```python
from build123d import *

# Parameters (mm, degrees)
SKETCH053_R         = 4
PAD024_DEPTH        = 134.8
SKETCH063_R         = 3.3
PAD028_DEPTH        = 8
SKETCH064_R         = 4
PAD029_DEPTH        = 50
CYLINDER001_R       = 100
CYLINDER001_DEPTH   = 100
CYLINDER001_FACE6_R = 4
PAD032_DEPTH        = 1.5
CYLINDER002_R       = 3.3
CYLINDER002_DEPTH   = 8


with BuildPart() as part:
    # Sketch053 (on Face1 of ShapeBinder012) → Pad024 (new body)
    with BuildSketch(Plane.YZ.offset(59.8)):
        with Locations((0, 75)):
            Circle(SKETCH053_R)
    extrude(amount=-PAD024_DEPTH)

    # Sketch063 (on Face3 of Pad024) → Pad028 (join)
    with BuildSketch(Plane(origin=(-75, 0, 0), x_dir=(0, -1, 0), z_dir=(-1, 0, 0))):
        with Locations((0, 75)):
            Circle(SKETCH063_R)
    extrude(amount=PAD028_DEPTH)

    # Sketch064 (on Face2 of Pad028) → Pad029 (join)
    with BuildSketch(Plane.YZ.offset(59.8)):
        with Locations((0, 75)):
            Circle(SKETCH064_R)
    extrude(amount=PAD029_DEPTH)

    # Cylinder001 → Cylinder001 (cut)
    with BuildSketch(Plane(origin=(83.8, 0, 75), x_dir=(0, -1, 0), z_dir=(1, 0, 0))):
        Circle(CYLINDER001_R)
    extrude(amount=CYLINDER001_DEPTH, mode=Mode.SUBTRACT)

    # Cylinder001 Face6 → Pad032 (add)
    with BuildSketch(Plane(origin=(83.8, 0, 75), x_dir=(0, -1, 0), z_dir=(1, 0, 0))):
        Circle(CYLINDER001_FACE6_R)
    extrude(amount=PAD032_DEPTH)

    # Cylinder002 → Cylinder002 (join)
    with BuildSketch(Plane(origin=(85.3, 0, 75), x_dir=(0, -1, 0), z_dir=(1, 0, 0))):
        Circle(CYLINDER002_R)
    extrude(amount=CYLINDER002_DEPTH)


solid = part.part
```
Can you work these out from the model? Positions are in its coordinate system, mm. A direction names the side the tool comes from. Coordinates: 2 decimals unless noted, no trailing zeros. Order: outer loops, then holes, each group sorted by start corner. A loop starts at its lowest first (then second) coordinate and runs counter-clockwise, first axis right, second up. Notation, with made-up numbers: (30.5, -35) - (35.5, -35) arc R29 cw to (35.5, -3) - close; hole circle Ø2 at (14, 76). An arc over 180 degrees is marked (long way). Answer in a Markdown table with one row per item.
1. Suppose I cut it at A-A (z = 75). Please give me the cut outline in (x, y), and give its area (3 significant figures).
Reply:
| item | result |
|---|---|
| outline | (-83, -3.3) - (-75, -3.3) - (-75, -4) - (85.3, -4) - (85.3, -3.3) - (93.3, -3.3) - (93.3, 3.3) - (85.3, 3.3) - (85.3, 4) - (-75, 4) - (-75, 3.3) - (-83, 3.3) - close |
| area | 1,390 mm^2 |
2. Suppose I cut it at B-B (y = 0). Please give me the cut outline in (x, z).
Reply:
| item | result |
|---|---|
| outline | (-83, 71.7) - (-75, 71.7) - (-75, 71) - (85.3, 71) - (85.3, 71.7) - (93.3, 71.7) - (93.3, 78.3) - (85.3, 78.3) - (85.3, 79) - (-75, 79) - (-75, 78.3) - (-83, 78.3) - close |
3. If I drill on line 1 along X through (y, z) = (3.5, 76.75); line 2 along Z through (x, y) = (-19, -2.25); line 3 along Z through (x, y) = (-48, 0.75), over which ranges is the centre line in solid material (lowest first)?
Reply:
| item | result |
|---|---|
| line 1 | x = -75 to 85.3 |
| line 2 | z = 71.69 to 78.31 |
| line 3 | z = 71.07 to 78.93 |
4. Suppose I cut it at C-C (x = 34). Please give me the cut outline in (y, z), and give its area (3 significant figures).
Reply:
| item | result |
|---|---|
| outline | circle Ø8 at (0, 75) |
| area | 50.3 mm^2 |
5. For faces 1 (the flat face through (-75, -2, 78)), 2 (the flat face through (-83, 0, 75)), 3 (the cylindrical face through (89.244, -1.774, 72.217)), which set-ups out of +Z, -Z, +X, -X, +Y, -Y let a thin tool reach every point of the face, with its end or its side?
Reply:
| item | result |
|---|---|
| face 1 | -X |
| face 2 | +Z, -Z, -X, +Y, -Y |
| face 3 | +X |
6. For pin 1 (1.5 mm diameter, centred on x = -36.5, z = 72, fed in from +Y); pin 2 (4 mm diameter, centred on x = -21.5, z = 72.5, fed in from -Y); pin 3 (1.5 mm diameter, centred on x = 29.5, y = 3, fed in from -Z), each with a flat end and sliding along its axis, tell me the tip position at first contact or that it passes through.
Reply:
| item | result |
|---|---|
| pin 1 | stops at y = 3.31 |
| pin 2 | stops at y = -3.97 |
| pin 3 | stops at z = 71.69 |
